For this review, take the finished solid that the model builds, in its own axes (mm). A direction names the side the tool comes from. Give positions to 0.01 mm unless a question says otherwise; leave off trailing zeros.
Q1. Insertion check: P1, Ø6, axis at y = 30, z = 17, coming from the +X side; P2, Ø8, axis at y = 16.5, z = 12.5, coming from the +X side; P3, Ø4.5, axis at x = 147, y = 47, coming from the -Z side. Each pin has a flat end and moves straight along its axis. Give the tip position at first contact, or say it passes through.
Q2. For line 1 (Y direction, x = 147, z = 2); line 2 (Y direction, x = 147, z = 6.5); line 3 (X direction, y = 49, z = 4.5), list the stretches that pass through material, from the lowest coordinate up.
Q3. Mouldability with a two-part tool opening along Y and no side actions: class faces 1 (the flat face through (147, 47, 10)), 2 (the flat face through (96, 48, 0)), 3 (the cylindrical face through (74.558, 3.002, 5.386)), 4 (the cylindrical face through (76.589, 90.945, 5.386)) as released by +Y, released by -Y, zero draft, split by the parting line, or undercut.
Q4. Machinability: for faces 5 (the flat face through (86, 47, 20)), 6 (the cylindrical face through (144.69, 46.04, 4.93)), 7 (the flat face through (0, 46, 8)), 8 (the cylindrical face through (74.282, 21.411, 19.524)), 9 (the cylindrical face through (76.307, 72.536, 19.524)), which of the approach directions +Z, -Z, +X, -X, +Y, -Y give a long, thin tool a straight path to every point of the face, cutting with its end or side? Answer none if there is none.
```python
from build123d import *
from OCP.BRepFilletAPI import BRepFilletAPI_MakeChamfer

# Parameters (mm, degrees)
EXTRUDE_1_DEPTH     = 20
CUT_EXTRUDE_1_DEPTH = 215.709105536
CHAMFER_1_SIZE      = 14
CHAMFER_1_SIZE2     = 19.269346887
FILLET_1_R          = 10
FILLET_2_R          = 3
SKETCH_3_R          = 2.5
CUT_EXTRUDE_2_DEPTH = 10


with BuildPart() as part:
    # ｽｹｯﾁ1 → 押し出し1 (new body)
    with BuildSketch(Plane.XY):
        Polygon((0, 0), (0, 94), (192, 89), (192, 5), align=None)
    extrude(amount=EXTRUDE_1_DEPTH)

    # ｽｹｯﾁ2 → ｶｯﾄ - 押し出し1 (cut, through all)
    with BuildSketch(Plane.XY.offset(20)):
        with BuildLine():
            Line((192, 89), (148.123504516, 90.14261707))
            ThreePointArc((148.123504516, 90.14261707), (177.911446327, 77.116941346), (190.157243541, 47))
            ThreePointArc((190.157243541, 47), (177.911447055, 16.883059402), (148.123506603, 3.857382984))
            Line((148.123506603, 3.857382984), (192, 5))
            Line((192, 5), (192, 89))
        make_face()
    extrude(amount=-CUT_EXTRUDE_1_DEPTH, mode=Mode.SUBTRACT)

    # 面取り1: one chamfer whose edges measure the first distance from different faces: ONE call of the kernel's chamfer builder (chamfer() names one face for all edges)
    chamfer_1_edges_1 = [part.edges().sort_by_distance(p)[0] for p in [
        (74.061752258, 92.071308535, 20),
    ]]
    chamfer_1_side_1 = [part.faces().sort_by_distance(p)[0] for p in [
        (74.061752258, 92.071308535, 10),
    ]]
    chamfer_1_edges_2 = [part.edges().sort_by_distance(p)[0] for p in [
        (190.157243541, 47.000001044, 20),
    ]]
    chamfer_1_side_2 = [part.faces().sort_by_distance(p)[0] for p in [
        (190.157243541, 47.000001044, 10),
    ]]
    chamfer_1_edges_3 = [part.edges().sort_by_distance(p)[0] for p in [
        (74.061753301, 1.928691492, 20),
    ]]
    chamfer_1_side_3 = [part.faces().sort_by_distance(p)[0] for p in [
        (74.061753301, 1.928691492, 10),
    ]]
    chamfer_1 = BRepFilletAPI_MakeChamfer(part.part.solid().wrapped)
    for e in chamfer_1_edges_1:
        chamfer_1.Add(CHAMFER_1_SIZE, CHAMFER_1_SIZE2, e.wrapped, chamfer_1_side_1[0].wrapped)  # the first distance lies on this face
    for e in chamfer_1_edges_2:
        chamfer_1.Add(CHAMFER_1_SIZE, CHAMFER_1_SIZE2, e.wrapped, chamfer_1_side_2[0].wrapped)  # the first distance lies on this face
    for e in chamfer_1_edges_3:
        chamfer_1.Add(CHAMFER_1_SIZE, CHAMFER_1_SIZE2, e.wrapped, chamfer_1_side_3[0].wrapped)  # the first distance lies on this face
    add(Compound.cast(chamfer_1.Shape()), mode=Mode.REPLACE)

    # ﾌｨﾚｯﾄ1
    fillet_1_edges = [part.edges().sort_by_distance(p)[0] for p in [
        (73.810934338, 72.801960541, 20),
        (170.887896654, 47.000000578, 20),
        (73.810935381, 21.198039486, 20),
        (74.061753301, 1.928691492, 6),
        (190.157243541, 47.000001044, 6),
        (74.061752258, 92.071308535, 6),
    ]]
    fillet(fillet_1_edges, radius=FILLET_1_R)

    # ﾌｨﾚｯﾄ2
    fillet_2_edges = [part.edges().sort_by_distance(p)[0] for p in [
        (0, 47, 20),
        (0, 10.38493898, 13.542542696),
        (0, 0, 0.452372753),
        (0, 83.61506102, 13.542542696),
        (0, 94, 0.452372753),
        (0, 92.909567354, 5.44490235),
        (0, 74.564948876, 19.510594551),
        (0, 1.090432646, 5.44490235),
        (0, 19.435051124, 19.510594551),
    ]]
    fillet(fillet_2_edges, radius=FILLET_2_R)

    # ｽｹｯﾁ3 → ｶｯﾄ - 押し出し2 (cut)
    with BuildSketch(Plane(origin=(0, 0, 0), x_dir=(-1, 0, 0), z_dir=(0, 0, -1))):
        with Locations((-147, 47)):
            Circle(SKETCH_3_R)
    extrude(amount=-CUT_EXTRUDE_2_DEPTH, mode=Mode.SUBTRACT)


solid = part.part
```
Computed:
1. P1: stops at x = 174.61
1. P2: stops at x = 173.6
1. P3: stops at z = 10
2. line 1: y = 3.89 to 44.5, 49.5 to 90.11
2. line 2: y = 5.54 to 44.5, 49.5 to 88.46
2. line 3: x = 0 to 145.5, 148.5 to 189.44
3. face 1: undercut
3. face 2: zero draft
3. face 3: released by -Y
3. face 4: released by +Y
4. face 5: +Z, +X, -X, +Y, -Y
4. face 6: -Z
4. face 7: +Z, -Z, -X, +Y, -Y
4. face 8: +Z, +X, -Y
4. face 9: +Z, +X, +Y
